Source: three-view drawing plus pictorial views. Frame: mm from the lowest corner of the part. Give positions to 0.01 mm unless a question says otherwise; leave off trailing zeros. Order: outer loops, then holes, each group sorted by start corner. A loop starts at its lowest first (then second) coordinate and runs counter-clockwise, first axis right, second up. Notation, with made-up numbers: (-30, 56.25) -> (11, 56.25) arc R33 cw to (11, 89.25) -> close; hole circle Ø5 at (65.5, -6.75). An arc over 180 degrees is marked (long way). Use a Markdown table: item, result. Add a question column.
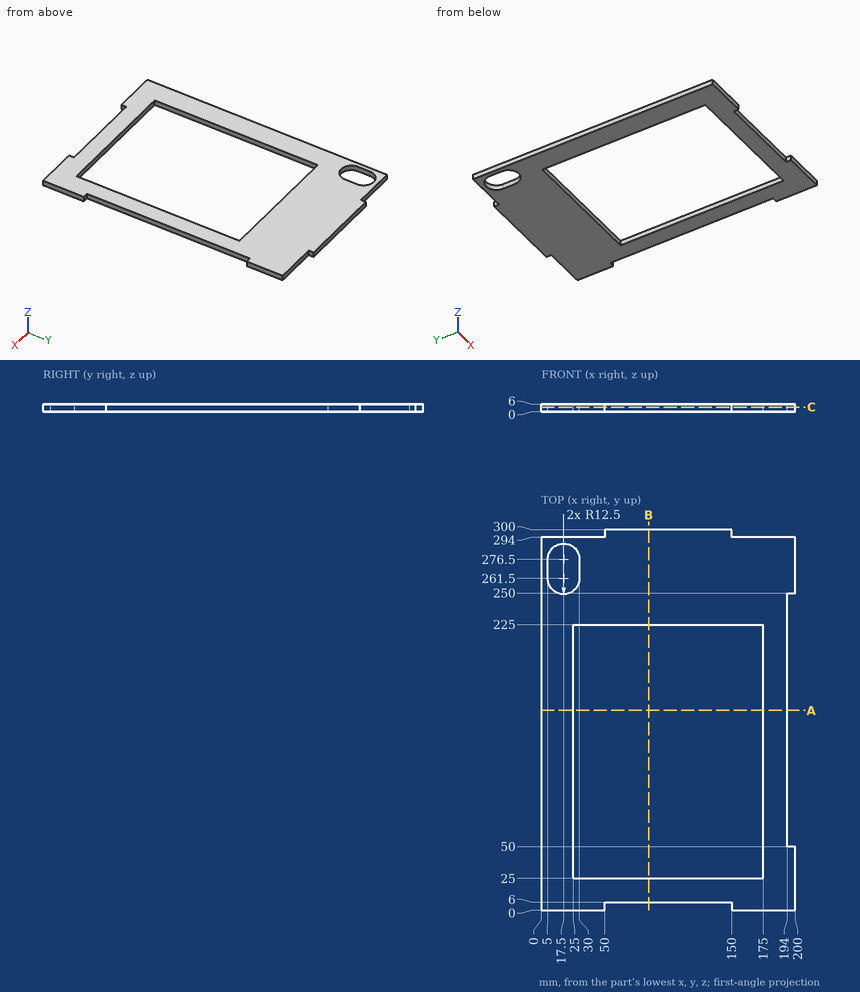
Q1. Ray query, line 1 (X direction, y = 91, z = 3.4); line 2 (Y direction, x = 153, z = 2); line 3 (X direction, y = 32.5, z = 1.95). Return the intervals inside material, ascending.
Q2. Section query C-C (z = 3.6). Return loops of the section in (x, y), plus the area to 3 significant figures.
Q3. Section query B-B (x = 84.5). Return loops of the section in (y, z).
Q4. Section query A-A (y = 157.5). Return loops of the section in (x, z).
Q5. First-contact query: pin 1 (1.8 mm diameter, centred on x = 128, z = 2.5, fed in from -Y); pin 2 (3 mm diameter, centred on x = 196.5, z = 3, fed in from +Y); pin 3 (3 mm diameter, centred on y = 132, z = 3.5, fed in from +X). Flat tips, straight axial feed; report the tip coordinate or a pass-through.
Solution:
| question | item | result |
|---|---|---|
| 1 | line 1 | x = 0 to 25, 175 to 194 |
| 1 | line 2 | y = 0 to 25, 225 to 294 |
| 1 | line 3 | x = 0 to 25, 175 to 200 |
| 2 | outline | (0, 0) -> (50, 0) -> (50, 6) -> (150, 6) -> (150, 0) -> (200, 0) -> (200, 50) -> (194, 50) -> (194, 250) -> (200, 250) -> (200, 294) -> (150, 294) -> (150, 300) -> (50, 300) -> (50, 294) -> (0, 294) -> close; hole (5, 261.5) arc R12.5 ccw to (30, 261.5) -> (30, 276.5) arc R12.5 ccw to (5, 276.5) -> close; hole (25, 25) -> (175, 25) -> (175, 225) -> (25, 225) -> close |
| 2 | area | 26,700 mm² |
| 3 | outline | (6, 0) -> (25, 0) -> (25, 6) -> (6, 6) -> close; (225, 0) -> (300, 0) -> (300, 6) -> (225, 6) -> close |
| 4 | outline | (0, 0) -> (25, 0) -> (25, 6) -> (0, 6) -> close; (175, 0) -> (194, 0) -> (194, 6) -> (175, 6) -> close |
| 5 | pin 1 | stops at y = 6 |
| 5 | pin 2 | stops at y = 294 |
| 5 | pin 3 | stops at x = 194 |
